```python
from build123d import *

# Parameters (mm, degrees)
SKETCH1_R           = 2.946896199
BOSS_EXTRUDE1_DEPTH = 1.5
SKETCH2_R           = 1.15
CUT_EXTRUDE1_DEPTH  = 1.5
SKETCH3_R           = 5.446896199
SKETCH3_R_2         = 2.946896199
BOSS_EXTRUDE2_DEPTH = 7
SKETCH4_R           = 4.25
BOSS_EXTRUDE3_DEPTH = 3
FILLET1_R           = 4
FILLET2_R           = 0.5
FILLET3_R           = 0.2


with BuildPart() as part:
    # Sketch1 → Boss-Extrude1 (new body)
    with BuildSketch(Plane(origin=(0, 0, 0), x_dir=(1, 0, 0), z_dir=(0, 1, 0))):
        with BuildLine():
            ThreePointArc((-4.043822449, -4.5), (0, -6.05), (4.043822449, -4.5))
            ThreePointArc((4.043822449, -4.5), (5.414156345, -3.625965374), (6.993227337, -3.240885753))
            ThreePointArc((6.993227337, -3.240885753), (10, 0), (6.993227337, 3.240885753))
            ThreePointArc((6.993227337, 3.240885753), (5.414156345, 3.625965374), (4.043822449, 4.5))
            ThreePointArc((4.043822449, 4.5), (0, 6.05), (-4.043822449, 4.5))
            ThreePointArc((-4.043822449, 4.5), (-5.414156345, 3.625965374), (-6.993227337, 3.240885753))
            ThreePointArc((-6.993227337, 3.240885753), (-10, 0), (-6.993227337, -3.240885753))
            ThreePointArc((-6.993227337, -3.240885753), (-5.414156345, -3.625965374), (-4.043822449, -4.5))
        make_face()
        with Locations(Location((0, 0, 0), (0, 0, 270))):
            Circle(SKETCH1_R, mode=Mode.SUBTRACT)
    extrude(amount=BOSS_EXTRUDE1_DEPTH)

    # Sketch2 → Cut-Extrude1 (cut)
    with BuildSketch(Plane(origin=(0, 1.5, 0), x_dir=(1, 0, 0), z_dir=(0, 1, 0))):
        with Locations(Location((-6.75, 0, 0), (0, 0, 270))):
            Circle(SKETCH2_R)
        with Locations(Location((6.75, 0, 0), (0, 0, 270))):
            Circle(SKETCH2_R)
    extrude(amount=-CUT_EXTRUDE1_DEPTH, mode=Mode.SUBTRACT)

    # Sketch3 → Boss-Extrude2 (add)
    with BuildSketch(Plane(origin=(0, 1.5, 0), x_dir=(1, 0, 0), z_dir=(0, 1, 0))):
        with Locations(Location((0, 0, 0), (0, 0, 270))):
            Circle(SKETCH3_R)
        with Locations(Location((0, 0, 0), (0, 0, 270))):
            Circle(SKETCH3_R_2, mode=Mode.SUBTRACT)
    extrude(amount=BOSS_EXTRUDE2_DEPTH)

    # Sketch4 → Boss-Extrude3 (add)
    with BuildSketch(Plane(origin=(0, 8.5, 0), x_dir=(1, 0, 0), z_dir=(0, 1, 0))):
        with Locations(Location((0, 0, 0), (0, 0, 270))):
            Circle(SKETCH4_R)
    extrude(amount=BOSS_EXTRUDE3_DEPTH)

    # Fillet1
    # the kernel refuses this fillet: 4 mm, written as the material it takes off along each edge
    with BuildSketch(Plane(origin=(0, 11.5, 0), x_dir=(0, 0, 1), z_dir=(-1, 0, 0))) as fillet1_piece_1:
        with BuildLine():
            CenterArc((0.377016654, -4), FILLET1_R, 14.477512186, 75.522487814)
            Line((0.377016654, 0), (0.377016654, 0.08))
            Line((0.377016654, 0.08), (4.25, 0.08))
            Line((4.25, 0.08), (4.33, 0))
            ThreePointArc((4.33, 0), (4.33, -1.5), (4.327459667, -2.98))
            Line((4.327459667, -2.98), (4.25, -3))
        make_face()
    revolve(axis=Axis((0, 11.5, 0), (0, 1, 0)), mode=Mode.SUBTRACT)

    # Fillet2
    fillet2_edges = [part.edges().sort_by_distance(p)[0] for p in [
        (0, 8.5, -5.446896199),
    ]]
    fillet(fillet2_edges, radius=FILLET2_R)

    # Fillet3
    fillet3_edges = [part.edges().sort_by_distance(p)[0] for p in [
        (0, 1.5, -5.446896199),
    ]]
    fillet(fillet3_edges, radius=FILLET3_R)


solid = part.part
```
Work out the finished part from the listing and answer in its coordinate system (mm). A direction names the side the tool comes from. Round coordinates to 2 decimals unless told otherwise and drop trailing zeros. Loops run counter-clockwise (first coordinate to the right, second up) from the corner with the lowest first, then second, coordinate; pieces in that order, holes last. Notation, with made-up numbers: M 59,39.25 L 117,39.25 A19 cw 117,45.25 Z; hole C 81.5,-9 d7. An arc over 180 degrees is marked long. Use CSV: the item, a comma, the result in double quotes.
Q1. Consider L1, parallel to X at y = 5.5, z = 0; L2, parallel to Y at x = 1.5, z = -5.5; L3, parallel to Z at x = 6.75, y = 1.05. Determine where each line is inside the solid, lowest interval first.
Determined:
L1,"-5.45 to -2.95, 2.95 to 5.45"
L2,"0 to 1.5"
L3,"-3.27 to -1.15, 1.15 to 3.27"
Q2. Section C-C, the plane x = -6.75 is taken. Determine the outline of the cut face in (y, z).
Determined:
outline,"M 0,-3.27 L 1.5,-3.27 L 1.5,-1.15 L 0,-1.15 Z; M 0,1.15 L 1.5,1.15 L 1.5,3.27 L 0,3.27 Z"
Q3. A tool of negligible diameter and unlimited length cuts with its end or side. For faces 1 (the flat face through (2, 0, 3)), 2 (the cylindrical face through (1.636, 4.801, 5.195)), 3 (the flat face through (0, 8.5, 0)), from which of +Z, -Z, +X, -X, +Y, -Y can it reach the whole face along a straight path? Write none if from no direction.
Determined:
face 1,"+Z, -Z, +X, -X, -Y"
face 2,"+Y"
face 3,"-Y"
Q4. Section A-A, the plane y = 3 is taken. Determine the outline of the cut face in (x, z), then the cut area to 3 significant figures.
Determined:
outline,"C 0,0 d10.89; hole C 0,0 d5.89"
area,"65.9 mm2"
Q5. Each of these flat-tipped pins is pushed along its axis until it touches: pin 1 (6 mm diameter, centred on y = 7, z = -2, fed in from +X); pin 2 (6 mm diameter, centred on y = 5, z = 4, fed in from -X); pin 3 (6 mm diameter, centred on x = 5, z = -1, fed in from +Y). Where does it stop, or does it pass through?
Determined:
pin 1,"x = 5.45"
pin 2,"x = -5.35"
pin 3,"y = 11.11"
Q6. Section B-B, the plane x = 7.5 is taken. Determine the outline of the cut face in (y, z), then the cut area to 3 significant figures.
Determined:
outline,"M 0,-3.16 L 1.5,-3.16 L 1.5,-0.87 L 0,-0.87 Z; M 0,0.87 L 1.5,0.87 L 1.5,3.16 L 0,3.16 Z"
area,"6.87 mm2"
Q7. The mould has two halves that part along X. Classify faces 4 (the cylindrical face through (10, 1, 0)), 5 (the flat face through (4, 8.5, 2)), 6 (the cylindrical face through (-5.393, 0.74, -3.635)), 7 (the cylindrical face through (7.89, 0.76, -0.15)): pulls with the +X half, pulls with the -X half, needs draft (parallel to the pull), parting line crosses it, or undercut.
Determined:
face 4,"pulls with the +X half"
face 5,"needs draft"
face 6,"pulls with the -X half"
face 7,"undercut"
